from build123d import *

# Parameters (mm, degrees)
SKETCH1_R           = 40
BOSS_EXTRUDE1_DEPTH = 1
SKETCH3_W           = 2.5
SKETCH3_H           = 80
BOSS_EXTRUDE2_DEPTH = 1


with BuildPart() as part:
    # Sketch1 → Boss-Extrude1 (new body)
    with BuildSketch(Plane.XY):
        with BuildLine():
            Line((-40, 50), (40, 50))
            ThreePointArc((40, 50), (47.071067812, 47.071067812), (50, 40))
            Line((50, 40), (50, -40))
            ThreePointArc((50, -40), (47.071067812, -47.071067812), (40, -50))
            Line((40, -50), (-40, -50))
            ThreePointArc((-40, -50), (-47.071067812, -47.071067812), (-50, -40))
            Line((-50, -40), (-50, 40))
            ThreePointArc((-50, 40), (-47.071067812, 47.071067812), (-40, 50))
        make_face()
        Circle(SKETCH1_R, mode=Mode.SUBTRACT)
    extrude(amount=BOSS_EXTRUDE1_DEPTH)

    # Sketch3 → Boss-Extrude2 (add)
    with BuildSketch(Plane.XY.offset(1)):
        with Locations((-33.75, 0)):
            Rectangle(SKETCH3_W, SKETCH3_H)
        with Locations((-26.25, 0)):
            Rectangle(SKETCH3_W, SKETCH3_H)
        with Locations((-18.75, 0)):
            Rectangle(SKETCH3_W, SKETCH3_H)
        with Locations((-11.25, 0)):
            Rectangle(SKETCH3_W, SKETCH3_H)
        with Locations((-3.75, 0)):
            Rectangle(SKETCH3_W, SKETCH3_H)
        with Locations((3.75, 0)):
            Rectangle(SKETCH3_W, SKETCH3_H)
        with Locations((11.25, 0)):
            Rectangle(SKETCH3_W, SKETCH3_H)
        with Locations((18.75, 0)):
            Rectangle(SKETCH3_W, SKETCH3_H)
        with Locations((26.25, 0)):
            Rectangle(SKETCH3_W, SKETCH3_H)
        with Locations((33.75, 0)):
            Rectangle(SKETCH3_W, SKETCH3_H)
    extrude(amount=-BOSS_EXTRUDE2_DEPTH)


solid = part.part
Check sheet for the modelled part. Datum: model origin and axes. Units: mm. Round coordinates to 2 decimals unless told otherwise and drop trailing zeros. Order: outer loops, then holes, each group sorted by start corner. A loop starts at its lowest first (then second) coordinate and runs counter-clockwise, first axis right, second up.
(1) Cross-section at A-A, the plane y = 32.5. State how many separate pieces and enclosed holes the cut face has, and give its area (3 significant figures).
(2) Draft check along Y on faces 1 (the cylindrical face through (40, -0.3, 0.5)), 2 (the cylindrical face through (-46.99, -47.15, 0.49)), 3 (the cylindrical face through (-47.15, 46.99, 0.49)). Enter one of: pulls with the +Y half, pulls with the -Y half, needs draft (parallel to the pull), parting line crosses it, or undercut.
(3) Scan lines: probe 1 along X at (y, z) = (-37, 0.2); probe 2 along Y at (x, z) = (-37, 0.45); probe 3 along Y at (x, z) = (32, 0.1). Record each from-to range of solid material in increasing order.
(4) Cross-section at B-B, the plane x = 14. Enter the section's corners in (y, z).
Check sheet entries:
1. separate pieces: 8
1. enclosed holes: 0
1. area: 68.4 mm2
2. face 1: undercut
2. face 2: pulls with the -Y half
2. face 3: pulls with the +Y half
3. probe 1: x = -50 to -15.2, -12.5 to -10, -5 to -2.5, 2.5 to 5, 10 to 12.5, 15.2 to 50
3. probe 2: y = -50 to -15.2, 15.2 to 50
3. probe 3: y = -50 to -24, 24 to 50
4. outline: (-50, 0) - (-37.47, 0) - (-37.47, 1) - (-50, 1) - close; (37.47, 0) - (50, 0) - (50, 1) - (37.47, 1) - close
